from build123d import *

# Parameters (mm, degrees)
SKETCH_1_R          = 16
SKETCH_1_R_2        = 4
SKETCH_1_R_3        = 1.5
EXTRUDE_1_DEPTH     = 4
SKETCH_2_R          = 7
SKETCH_2_R_2        = 4
EXTRUDE_2_DEPTH     = 10
SKETCH_3_R          = 1.5
CUT_EXTRUDE_1_DEPTH = 10
SKETCH_4_R          = 1.5
CUT_EXTRUDE_2_DEPTH = 10


with BuildPart() as part:
    # 草图1 → 凸台-拉伸1 (new body)
    with BuildSketch(Plane.XY):
        Circle(SKETCH_1_R)
        Circle(SKETCH_1_R_2, mode=Mode.SUBTRACT)
        with Locations((0, -11.5)):
            Circle(SKETCH_1_R_3, mode=Mode.SUBTRACT)
        with Locations((-9.959292144, -5.75)):
            Circle(SKETCH_1_R_3, mode=Mode.SUBTRACT)
        with Locations((-9.959292144, 5.75)):
            Circle(SKETCH_1_R_3, mode=Mode.SUBTRACT)
        with Locations((0, 11.5)):
            Circle(SKETCH_1_R_3, mode=Mode.SUBTRACT)
        with Locations((9.959292144, 5.75)):
            Circle(SKETCH_1_R_3, mode=Mode.SUBTRACT)
        with Locations((9.959292144, -5.75)):
            Circle(SKETCH_1_R_3, mode=Mode.SUBTRACT)
    extrude(amount=EXTRUDE_1_DEPTH)

    # 草图2 → 凸台-拉伸2 (add)
    with BuildSketch(Plane.XY.offset(4)):
        Circle(SKETCH_2_R)
        Circle(SKETCH_2_R_2, mode=Mode.SUBTRACT)
    extrude(amount=EXTRUDE_2_DEPTH)

    # 草图3 → 切除-拉伸1 (cut)
    with BuildSketch(Plane(origin=(0, 0, 0), x_dir=(1, 0, 0), z_dir=(0, 1, 0))):
        with Locations(Location((0, -9, 0), (0, 0, 270))):
            Circle(SKETCH_3_R)
    extrude(amount=-CUT_EXTRUDE_1_DEPTH, mode=Mode.SUBTRACT)

    # 草图4 → 切除-拉伸2 (cut)
    with BuildSketch(Plane(origin=(0, 0, 0), x_dir=(0, 0, -1), z_dir=(1, 0, 0))):
        with Locations(Location((-9, 0, 0), (0, 0, 180))):
            Circle(SKETCH_4_R)
    extrude(amount=-CUT_EXTRUDE_2_DEPTH, mode=Mode.SUBTRACT)


solid = part.part
CAD build for the part. Positions are in the model's coordinates, mm. A direction names the side the tool comes from. Give positions to 0.01 mm unless a question says otherwise; leave off trailing zeros. Write each loop counter-clockwise with the first axis right and the second up, starting at its lowest first coordinate (ties: lowest second). Pieces come first, ordered by that corner, then holes. Notation, with made-up numbers: M 7,7.5 L 29,7.5 A24 ccw 29,35.5 Z; hole C 52,-4.5 d6. An arc over 180 degrees is marked long. Put each result on its own line as item: value. Start each with the question number.
(1) Band-saw the part on C-C, the plane y = 0. Write the cut outline in (x, z), and give its area (3 significant figures).
(2) Band-saw the part on B-B, the plane x = 0. Write the cut outline in (y, z).
(3) Which spindle directions (+Z, -Z, +X, -X, +Y, -Y) get a long thin tool onto all of the face, cutting with end or side? Do faces 1 (the face through (0, -13, 2)), 2 (the face through (6.677, 2.103, 8.93)). Say none if no direction does.
(4) Flat gauge pins, fed straight in: pin 1 Ø5 at (x, y) = (-9.96, -5.75) entering from +Z; pin 2 Ø8 at (x, z) = (-3.5, 11.5) entering from +Y; pin 3 Ø6 at (x, y) = (-5, -11.5) entering from -Z; pin 4 Ø2 at (y, z) = (-6.5, 4) entering from +X (3 decimals). Where does each tip first touch, or does it go through?
(5) Probe L1, parallel to Y at x = 0, z = 1.35; L2, parallel to Z at x = 0, y = -5.9; L3, parallel to Y at x = -1, z = 3.5. List the from-to ranges inside material, lowest first.
(6) Band-saw the part on A-A, the plane y = -5. Write the cut outline in (x, z).
(7) Mould opens along Z. For faces 3 (the face through (-0.2, 7.3, 4)), 4 (the face through (-0.575, -5.333, 10.386)), 5 (the face through (-5.331, 0.575, 10.386)), 6 (the face through (-8.57, -6.32, 1.97)) say: +Z half, -Z half, draft (parallel to the pull), parting line (faces both ways), or undercut.
(8) Band-saw the part on D-D, the plane z = 9. Write the cut outline in (x, y), and give its area (3 significant figures).
Response values:
1. outline: M -16,0 L -4,0 L -4,7.5 L -7,7.5 L -7,4 L -16,4 Z; M -7,10.5 L -4,10.5 L -4,14 L -7,14 Z; M 4,0 L 16,0 L 16,4 L 7,4 L 7,14 L 4,14 Z
1. area: 147 mm2
2. outline: M -16,0 L -13,0 L -13,4 L -16,4 Z; M -10,0 L -4,0 L -4,7.5 L -7,7.5 L -7,4 L -10,4 Z; M -7,10.5 L -4,10.5 L -4,14 L -7,14 Z; M 4,0 L 10,0 L 10,4 L 7,4 L 7,14 L 4,14 Z; M 13,0 L 16,0 L 16,4 L 13,4 Z
3. face 1: +Z, -Z
3. face 2: +Z
4. pin 1: stops at z = 4
4. pin 2: stops at y = 7
4. pin 3: stops at z = 0
4. pin 4: stops at x = 15.025
5. L1: y = -16 to -13, -10 to -4, 4 to 10, 13 to 16
5. L2: z = 0 to 7.5, 10.5 to 14
5. L3: y = -15.97 to -12.62, -10.38 to -3.87, 3.87 to 10.38, 12.62 to 15.97
6. outline: M -15.2,0 L -11.26,0 L -11.26,4 L -15.2,4 Z; M -8.66,0 L 8.66,0 L 8.66,4 L 4.9,4 L 4.9,14 L -4.9,14 L -4.9,4 L -8.66,4 Z; M 11.26,0 L 15.2,0 L 15.2,4 L 11.26,4 Z; hole C 0,9 d3
7. face 3: +Z half
7. face 4: undercut
7. face 5: undercut
7. face 6: draft
8. outline: M -6.84,-1.5 A7 ccw -1.5,-6.84 L -1.5,-3.71 A4 cw -3.71,-1.5 Z; M -6.84,1.5 L -3.71,1.5 A4 cw long 1.5,-3.71 L 1.5,-6.84 A7 ccw long Z
8. area: 85.4 mm2
